Work out the finished part from the listing and answer in its coordinate system (mm). Face numbers are marked on the shaded views. A direction names the side the tool comes from. Coordinates: 2 decimals unless noted, no trailing zeros. Order: outer loops, then holes, each group sorted by start corner. A loop starts at its lowest first (then second) coordinate and runs counter-clockwise, first axis right, second up. Notation, with made-up numbers: M 52.5,1 L 86.5,1 A5 ccw 86.5,9 Z; hole C 26,-11.75 d7. An arc over 180 degrees is marked long. Use a Markdown table: item, result.
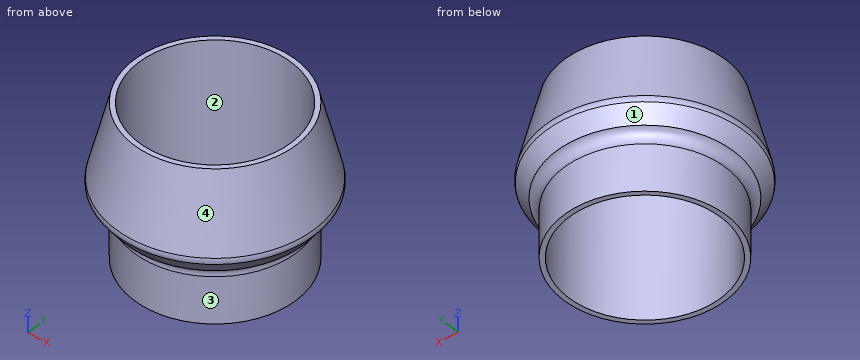
from build123d import *


with BuildPart() as part:
    # Esboço1 → Revolução4 (revolve)
    with BuildSketch(Plane(origin=(0, 0, 0), x_dir=(0, 0, -1), z_dir=(1, 0, 0)), mode=Mode.PRIVATE) as revolu_o4_sk:
        with BuildLine():
            Line((-36.699570276, 4.133360134), (-36.092161543, 3.695324027))
            ThreePointArc((-36.092161543, 3.695324027), (-35.905826449, 3.430249421), (-35.58663159, 3.374572178))
            Line((-35.58663159, 3.374572178), (-33.65, 3.374572178))
            Line((-33.65, 3.374572178), (-33.65, 3.175))
            Line((-33.65, 3.175), (-40, 3.175))
            Line((-40, 3.175), (-40, 3.3734375))
            Line((-40, 3.3734375), (-36.951032326, 4.135679419))
            ThreePointArc((-36.951032326, 4.135679419), (-36.825153111, 4.150586903), (-36.699570276, 4.133360134))
        make_face()
    revolve(revolu_o4_sk.sketch.rotate(Axis((0, 0, 40), (0, 0, -1)), 90), axis=Axis((0, 0, 40), (0, 0, -1)))


solid = part.part
1. Section C-C on z = 34 is taken. Determine the outline of the cut face in (x, y) (3 decimals), then the cut area to 3 significant figures.
Answers below:
| item | result |
|---|---|
| outline | C 0,0 d6.749; hole C 0,0 d6.35 |
| area | 4.11 mm² |
2. Section D-D on z = 39 is taken. Determine the outline of the cut face in (x, y) (3 decimals), then the cut area to 3 significant figures.
Answers below:
| item | result |
|---|---|
| outline | C 0,0 d7.247; hole C 0,0 d6.35 |
| area | 9.58 mm² |
3. For the marked faces 3 and 4, determine the directions among +Z, -Z, +X, -X, +Y, -Y from which every point of the face is accessible in a straight line to the end or side of a thin tool.
Answers below:
| item | result |
|---|---|
| face 3 | -Z |
| face 4 | +Z |
4. Flat-ended cylindrical pins translate along their axes: P1, Ø1.5, axis at x = 2.5, z = 35.5, coming from the -Y side; P2, Ø1, axis at x = -1.5, y = 2, coming from the +Z side. Find the tip coordinate at first contact, or state that the pin passes through.
Answers below:
| item | result |
|---|---|
| P1 | y = -3.08 |
| P2 | through |
5. Section A-A on x = 0 is taken. Determine the outline of the cut face in (y, z) (3 decimals).
Answers below:
| item | result |
|---|---|
| outline | M -4.136,36.951 A0.5 ccw -4.133,36.7 L -3.695,36.092 A0.423 cw -3.375,35.587 L -3.375,33.65 L -3.175,33.65 L -3.175,40 L -3.373,40 Z; M 3.175,33.65 L 3.375,33.65 L 3.375,35.587 A0.423 cw 3.695,36.092 L 4.133,36.7 A0.5 ccw 4.136,36.951 L 3.373,40 L 3.175,40 Z |
6. For a pull along Y with two mould halves and no side action, classify the marked faces 1 and 2 as +Y half, -Y half, draft (parallel to the pull), parting line (faces both ways), or undercut.
Answers below:
| item | result |
|---|---|
| face 1 | parting line |
| face 2 | undercut |
7. Find the intervals of material crossed by probe 1 along Y at (x, z) = (0, 37) (3 decimals); probe 2 along X at (y, z) = (-0.5, 38.75); probe 3 along Y at (x, z) = (0.5, 39), in increasing order.
Answers below:
| item | result |
|---|---|
| probe 1 | -4.123 to -3.175, 3.175 to 4.123 |
| probe 2 | -3.65 to -3.14, 3.14 to 3.65 |
| probe 3 | -3.59 to -3.14, 3.14 to 3.59 |
